from build123d import *

# Parameters (mm, degrees)
SKETCH1_R                       = 30
BOSS_EXTRUDE1_DEPTH             = 5
SKETCH8_R                       = 4.75
BOSS_EXTRUDE3_DEPTH             = 10
SKETCH9_R                       = 5.75
CUT_EXTRUDE3_DEPTH              = 4
SKETCH16_W                      = 21
SKETCH16_H                      = 16
BOSS_EXTRUDE7_DEPTH             = 10
BOSS_EXTRUDE7_DIRECTION_2_REACH = 62.052
SKETCH17_W                      = 21
SKETCH17_H                      = 2
BOSS_EXTRUDE8_DEPTH             = 20
SKETCH18_R                      = 3
CUT_EXTRUDE4_DEPTH              = 8


with BuildPart() as part:
    # Sketch1 → Boss-Extrude1 (new body)
    with BuildSketch(Plane(origin=(0, 0, 0), x_dir=(1, 0, 0), z_dir=(0, 1, 0))):
        with Locations(Location((0, 0, 0), (0, 0, 270))):
            Circle(SKETCH1_R)
    extrude(amount=BOSS_EXTRUDE1_DEPTH)

    # Sketch8 → Boss-Extrude3 (add)
    with BuildSketch(Plane(origin=(10, 0, 0), x_dir=(0, 0, -1), z_dir=(1, 0, 0))):
        with BuildLine():
            Line((-7.5, 0), (-7.5, -35))
            ThreePointArc((-7.5, -35), (0, -42.5), (7.5, -35))
            Line((7.5, -35), (7.5, 0))
            Line((7.5, 0), (-7.5, 0))
        make_face()
        with Locations((0, -35)):
            Circle(SKETCH8_R, mode=Mode.SUBTRACT)
    boss_extrude3 = extrude(amount=-BOSS_EXTRUDE3_DEPTH)

    # Sketch9 → Cut-Extrude3 (cut)
    with BuildSketch(Plane.ZY.offset(-10)):
        with Locations((0, -35)):
            Circle(SKETCH9_R)
    cut_extrude3 = extrude(amount=CUT_EXTRUDE3_DEPTH, mode=Mode.SUBTRACT)

    # Mirror1: Boss-Extrude3, Cut-Extrude3 across plane
    add(boss_extrude3.mirror(Plane(origin=(0, 0, 0), x_dir=(0, 0, 1), z_dir=(1, 0, 0))))
    add(cut_extrude3.mirror(Plane(origin=(0, 0, 0), x_dir=(0, 0, 1), z_dir=(1, 0, 0))), mode=Mode.SUBTRACT)

    # Sketch16 → Boss-Extrude7 (add)
    with BuildSketch(Plane(origin=(0, 0, 0), x_dir=(-1, 0, 0), z_dir=(0, -1, 0))):
        with Locations((35, 0)):
            Rectangle(SKETCH16_W, SKETCH16_H)
    extrude(amount=BOSS_EXTRUDE7_DEPTH)

    # Boss-Extrude7 direction 2: up to this face of the body (flat: up to its plane)
    boss_extrude7_direction_2_end = Plane(part.part.faces().sort_by_distance((0, 5, 0))[0])
    # Sketch16 → Boss-Extrude7 direction 2 (add, up to the picked face)
    with BuildSketch(Plane(origin=(0, 0, 0), x_dir=(-1, 0, 0), z_dir=(0, -1, 0)), mode=Mode.PRIVATE) as boss_extrude7_direction_2_sk1:
        with Locations((35, 0)):
            Rectangle(SKETCH16_W, SKETCH16_H)
    boss_extrude7_direction_2_tool1 = split(extrude(boss_extrude7_direction_2_sk1.sketch, amount=-BOSS_EXTRUDE7_DIRECTION_2_REACH, mode=Mode.PRIVATE), bisect_by=boss_extrude7_direction_2_end, keep=Keep.BOTH, mode=Mode.PRIVATE)
    add(boss_extrude7_direction_2_tool1.solids().sort_by(Axis((-35, 0, 0), (0, 1, 0)))[0])

    # Sketch17 → Boss-Extrude8 (add)
    with BuildSketch(Plane.XZ.offset(10)):
        with Locations((-35, 7)):
            Rectangle(SKETCH17_W, SKETCH17_H)
        with Locations((-35, -7)):
            Rectangle(SKETCH17_W, SKETCH17_H)
    extrude(amount=BOSS_EXTRUDE8_DEPTH)

    # Sketch18 → Cut-Extrude4 (cut)
    with BuildSketch(Plane(origin=(0, 5, 0), x_dir=(1, 0, 0), z_dir=(0, 1, 0))):
        with Locations(Location((0, 0, 0), (0, 0, 270))):
            Circle(SKETCH18_R)
    extrude(amount=-CUT_EXTRUDE4_DEPTH, mode=Mode.SUBTRACT)


solid = part.part
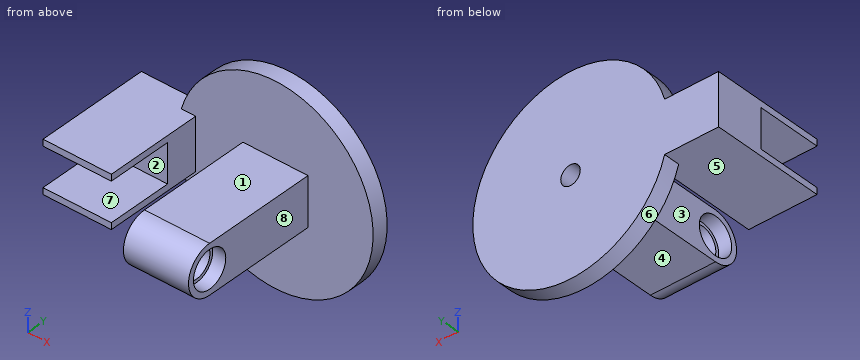
The model under review builds one solid part; all positions refer to its coordinate system, in mm. Face numbers are marked on the shaded views. A direction names the side the tool comes from. Coordinates: 2 decimals unless noted, no trailing zeros. Loops run counter-clockwise (first coordinate to the right, second up) from the corner with the lowest first, then second, coordinate; pieces in that order, holes last. Notation, with made-up numbers: M 41,-21.5 L 51,-21.5 A21 ccw 51,-2.5 Z; hole C 3,34 d4. An arc over 180 degrees is marked long. Put each result on its own line as item: value. Start each with the question number.
Q1. Add section C-C (x = 0). Write out the cut boundary in (y, z).
Q2. Add section B-B (z = 0). Write out the cut boundary in (x, y).
Q3. The part is to be moulded in two halves that separate along Z. For the marked faces 5, 6, 7 and 8, say which applies: +Z half, -Z half, draft (parallel to the pull), parting line (faces both ways), or undercut.
Q4. Add section D-D (y = -32.5). Write out the cut boundary in (x, z), and give its area (3 significant figures).
Q5. Wall thickness on line 1 (Z direction, x = 3, y = -35); line 2 (X direction, y = -0.5, z = -1); line 3 (Y direction, x = 0, z = 0): over which ranges is each line inside the solid? List them lowest first.
Q6. Clearance check with flat-ended pins moving along their axes: pin 1 (5 mm diameter, centred on x = -23, y = -8.5, fed in from -Z); pin 2 (10 mm diameter, centred on y = -37.5, z = 17, fed in from -X); pin 3 (4.5 mm diameter, centred on y = -26, z = -2, fed in from -X); pin 4 (0.6 mm diameter, centred on x = -36, z = -6.5, fed in from -Y). State where each tip first meets the part, or that it passes through.
Q7. Add section A-A (y = -12). Write out the cut boundary in (x, z).
Q8. For the marked faces 1, 2, 3 and 4, list the 3-axis set-ups (+Z, -Z, +X, -X, +Y, -Y) from which the entire face can be reached by the end or side of a thin tool; tool diameter is ignored.
Answers:
1. outline: M -35,-7.5 L 0,-7.5 L 0,-30 L 5,-30 L 5,-3 L -3,-3 L -3,3 L 5,3 L 5,30 L 0,30 L 0,7.5 L -35,7.5 A7.5 ccw Z; hole C -35,0 d9.5
2. outline: M -45.5,-10 L -24.5,-10 L -24.5,0 L -10,0 L -10,-29.25 L -6,-29.25 L -6,-30.25 L 6,-30.25 L 6,-29.25 L 10,-29.25 L 10,0 L 30,0 L 30,5 L 3,5 L 3,-3 L -3,-3 L -3,5 L -45.5,5 Z; M -10,-42.5 L 10,-42.5 L 10,-40.75 L 6,-40.75 L 6,-39.75 L -6,-39.75 L -6,-40.75 L -10,-40.75 Z
3. face 5: -Z half
3. face 6: parting line
3. face 7: undercut
3. face 8: draft
4. outline: M -10,-7.5 L 10,-7.5 L 10,-5.18 L 6,-5.18 L 6,-4.04 L -6,-4.04 L -6,-5.18 L -10,-5.18 Z; M -10,5.18 L -6,5.18 L -6,4.04 L 6,4.04 L 6,5.18 L 10,5.18 L 10,7.5 L -10,7.5 Z
4. area: 120 mm^2
5. line 1: z = -7.5 to -4.75, 4.75 to 7.5
5. line 2: x = -45.5 to -24.5, -10 to -2.83, 2.83 to 10
5. line 3: y = -42.5 to -39.75, -30.25 to -3
6. pin 1: stops at z = -8
6. pin 2: passes through
6. pin 3: stops at x = -10
6. pin 4: stops at y = -30
7. outline: M -45.5,-8 L -24.5,-8 L -24.5,-6 L -45.5,-6 Z; M -45.5,6 L -24.5,6 L -24.5,8 L -45.5,8 Z; M -10,-7.5 L 10,-7.5 L 10,7.5 L -10,7.5 Z
8. face 1: +Z, +X, -Y
8. face 2: -X, -Y
8. face 3: +Z, -Z, -Y
8. face 4: -Z, +X, -Y
